Autodesk Inventor part; units mm, degrees
ref_plane "YZ Plane" through (0, 0, 0) normal (1, 0, 0) x (0, 1, 0)
ref_plane "XZ Plane" through (0, 0, 0) normal (0, 1, 0) x (-1, 0, 0)
ref_plane "XY Plane" through (0, 0, 0) normal (0, 0, 1) x (1, 0, 0)
sketch "Sketch1" plane through (0, 0, 0) normal (0, 1, 0) x (-1, 0, 0)
  line L0 (0, 0) -> (0, -322.934) construction
  line L1 (5, 0) -> (5, -322.934)
  line L2 (-5, -322.934) -> (-5, 0)
  arc A0 (5, 0) -> (-5, 0) centre (0, 0) ccw
  arc A1 (-5, -322.934) -> (5, -322.934) centre (0, -322.934) ccw
  circle A2 centre (0, 0) radius 1.65
  circle A3 centre (0, -322.934) radius 1.65
  circle A4 centre (0, -74.182) radius 1.65
  circle A5 centre (0, -218.733) radius 1.65
  arc A6 (5, -74.182) -> (5, -218.733) centre (600.631, -146.4575) ccw
  arc A7 (-5, -74.182) -> (-5, -218.733) centre (590.631, -146.4575) ccw
  point P0 (0, -161.467)
  dimension "d0" = 3.3
  dimension "d1" = 3.3
  dimension "d2" = 10
  dimension "d3" = 322.934
  dimension "d4" = 3.3
  dimension "d5" = 74.182
  dimension "d8" = 3.3
  dimension "d9" = 218.733
  dimension "d12" = 600
  dimension "d13" = 600
extrude "Extrusion1" add sketch "Sketch1" along normal blind 3 contours L1 A6 A1 L2 A0 | L2 A7
Here's how the part is built. I have some questions about the finished solid (model axes, mm). Coordinates: 2 decimals unless noted, no trailing zeros. Order: outer loops, then holes, each group sorted by start corner. A loop starts at its lowest first (then second) coordinate and runs counter-clockwise, first axis right, second up.
1) I need wall thicknesses on line 1 (Z direction, x = 0, y = 1.5); line 2 (Z direction, x = -0.25, y = 2.15); line 3 (X direction, y = 2.15, z = -74). Which ranges of each line are inside material? Lowest first, please.
2) Imagine slicing it at B-B on z = -113.5. List the corners of the cut face in (x, y) for me.
3) Will these pins go through, and if not, where does the flat tip stop? pin 1 (3 mm diameter, centred on x = 0, z = -322.934, fed in from +Y); pin 2 (0.9 mm diameter, centred on y = 1, z = -265.5, fed in from +X).
4) Imagine slicing it at A-A on y = 2.4. List the corners of the cut face in (x, z) for me, and give its area (3 significant figures).
Response values:
1. line 1: z = -327.93 to -324.58, -321.28 to -220.38, -217.08 to -75.83, -72.53 to -1.65, 1.65 to 5
1. line 2: z = -327.93 to -324.56, -321.3 to -220.36, -217.1 to -75.81, -72.55 to -1.63, 1.63 to 4.99
1. line 3: x = -5 to -1.64, 1.64 to 5
2. outline: (-1.54, 0) - (8.46, 0) - (8.46, 3) - (-1.54, 3) - close
3. pin 1: passes through
3. pin 2: stops at x = 5
4. outline: (-5, -322.93) arc R5 ccw to (5, -322.93) - (5, -218.73) arc R600 ccw to (5, -74.18) - (5, 0) arc R5 ccw to (-5, 0) - (-5, -74.18) arc R600 cw to (-5, -218.73) - close; hole circle Ø3.3 at (0, -322.93); hole circle Ø3.3 at (0, -218.73); hole circle Ø3.3 at (0, -74.18); hole circle Ø3.3 at (0, 0)
4. area: 3,270 mm2
